```python
from build123d import *

# Parameters (mm, degrees)
SKETCH1_W           = 36.957
SKETCH1_H           = 21.3995
SKETCH1_R           = 1.190625
SKETCH1_R_2         = 0.9525
BOSS_EXTRUDE1_DEPTH = 2.38125
BOSS_EXTRUDE3_DEPTH = 2.38125
CUT_EXTRUDE2_REACH  = 4.381
SKETCH4_R           = 2.4892
FILLET1_R           = 2.54


with BuildPart() as part:
    # Sketch1 → Boss-Extrude1 (new body)
    with BuildSketch(Plane.XY):
        with Locations((16.891, 9.11225)):
            Rectangle(SKETCH1_W, SKETCH1_H)
        with Locations((1.5875, 14.25575)):
            Circle(SKETCH1_R, mode=Mode.SUBTRACT)
        with Locations((32.1945, 1.5875)):
            Circle(SKETCH1_R_2, mode=Mode.SUBTRACT)
    extrude(amount=BOSS_EXTRUDE1_DEPTH)

    # Sketch2 → Boss-Extrude3 (add)
    with BuildSketch(Plane.XZ.offset(1.5875)):
        Polygon((-1.5875, 2.38125), (35.3695, 2.38125), (35.3695, 0), (48.0695, -21.997045256), (31.571716058, -31.522045256), (13.372454744, 0), (-1.5875, 0), align=None)
    extrude(amount=BOSS_EXTRUDE3_DEPTH)

    # Sketch4 → Cut-Extrude2 (cut, up to next)
    with BuildSketch(Plane(origin=(0, -1.5875, 0), x_dir=(1, 0, 0), z_dir=(0, 1, 0)), mode=Mode.PRIVATE) as cut_extrude2_sk1:
        with Locations((35.800977372, 19.797340731)):
            Circle(SKETCH4_R)
    cut_extrude2_tool1 = extrude(cut_extrude2_sk1.sketch, amount=-CUT_EXTRUDE2_REACH, mode=Mode.PRIVATE) & part.part
    add(cut_extrude2_tool1.solids().sort_by_distance((35.800977, -1.5875, -19.797341))[0], mode=Mode.SUBTRACT)
    # Sketch4 → Cut-Extrude2 (cut, up to next)
    with BuildSketch(Plane(origin=(0, -1.5875, 0), x_dir=(1, 0, 0), z_dir=(0, 1, 0)), mode=Mode.PRIVATE) as cut_extrude2_sk2:
        with Locations((29.450977372, 8.798818102)):
            Circle(SKETCH4_R)
    cut_extrude2_tool2 = extrude(cut_extrude2_sk2.sketch, amount=-CUT_EXTRUDE2_REACH, mode=Mode.PRIVATE) & part.part
    add(cut_extrude2_tool2.solids().sort_by_distance((29.450977, -1.5875, -8.798818))[0], mode=Mode.SUBTRACT)

    # Fillet1
    fillet1_edges = [part.edges().sort_by_distance(p)[0] for p in [
        (24.370977372, -1.5875, 0),
    ]]
    fillet(fillet1_edges, radius=FILLET1_R)


solid = part.part
```
Source: CAD feature listing. Evaluate the final solid. Frame: model axes, mm. A direction names the side the tool comes from. Coordinates: 2 decimals unless noted, no trailing zeros. Write each loop counter-clockwise with the first axis right and the second up, starting at its lowest first coordinate (ties: lowest second). Pieces come first, ordered by that corner, then holes. Notation, with made-up numbers: (50.25, 47.5) - (68.25, 47.5) arc R16 cw to (68.25, 57.5) - close; hole circle Ø5 at (-8, -9). An arc over 180 degrees is marked (long way). Answer as a JSON object with one key per item and string values.
Q1. Section query B-B, the plane y = -2.5. Output: boundary loops of the cut face in (x, z), plus the area to 3 significant figures.
Ans:
{"outline": "(-1.59, 0) - (13.37, 0) - (31.57, -31.52) - (48.07, -22) - (35.37, 0) - (35.37, 2.38) - (-1.59, 2.38) - close; hole circle Ø4.98 at (29.45, -8.8); hole circle Ø4.98 at (35.8, -19.8)", "area": "638 mm2"}
Q2. Section query A-A, the plane x = 37.5. Output: boundary loops of the cut face in (y, z), plus the area to 3 significant figures.
Ans:
{"outline": "(-3.97, -28.1) - (-1.59, -28.1) - (-1.59, -21.62) - (-3.97, -21.62) - close; (-3.97, -17.98) - (-1.59, -17.98) - (-1.59, -3.69) - (-3.97, -3.69) - close", "area": "49.5 mm2"}
Q3. First-contact query: pin 1 Ø1.9 at (x, y) = (1.59, 14.26) entering from -Z (1 decimal); pin 2 Ø3 at (x, y) = (31, 1) entering from -Z; pin 3 Ø8 at (x, z) = (24.5, -15.5) entering from +Y; pin 4 Ø7 at (x, y) = (20.5, 7.5) entering from -Z. Flat tips, straight axial feed; report the tip coordinate or a pass-through.
Ans:
{"pin 1": "passes through", "pin 2": "stops at z = -0.46", "pin 3": "stops at y = -1.59", "pin 4": "stops at z = 0"}
Q4. Section query C-C, the plane x = 7. Output: boundary loops of the cut face in (y, z).
Ans:
{"outline": "(-3.97, 0) - (19.81, 0) - (19.81, 2.38) - (-3.97, 2.38) - close"}
Q5. Material intervals for line 1 (Z direction, x = 12, y = 15); line 2 (Y direction, x = 45.5, z = -21); line 3 (Z direction, x = 29, y = -2.25), sorted ascending. Write a range as [from, to].
Ans:
{"line 1": "z = [0, 2.38]", "line 2": "y = [-3.97, -1.59]", "line 3": "z = [-27.07, -11.25], [-6.35, 2.38]"}
Q6. Section query D-D, the plane y = 9.75. Output: boundary loops of the cut face in (x, z).
Ans:
{"outline": "(-1.59, 0) - (35.37, 0) - (35.37, 2.38) - (-1.59, 2.38) - close"}
Q7. Draft query along Y for faces 1 (the flat face through (35.37, 8, 1)), 2 (the flat face through (17, 19.812, 1)), 3 (the cylindrical face through (33.074, 1.223, 1.174)). Return one class per face: released by +Y, released by -Y, zero draft, split by the parting line, or undercut.
Ans:
{"face 1": "zero draft", "face 2": "released by +Y", "face 3": "undercut"}
Q8. Set-up query: faces 4 (the flat face through (32, -1.588, -14)), 5 (the flat face through (-1.588, 8, 1)). Return all of +Z, -Z, +X, -X, +Y, -Y with unobstructed straight access to the full face (end or side cutting, diameter ignored); none if empty.
Ans:
{"face 4": "-Z, +X, -X, +Y", "face 5": "+Z, -Z, -X, +Y, -Y"}
